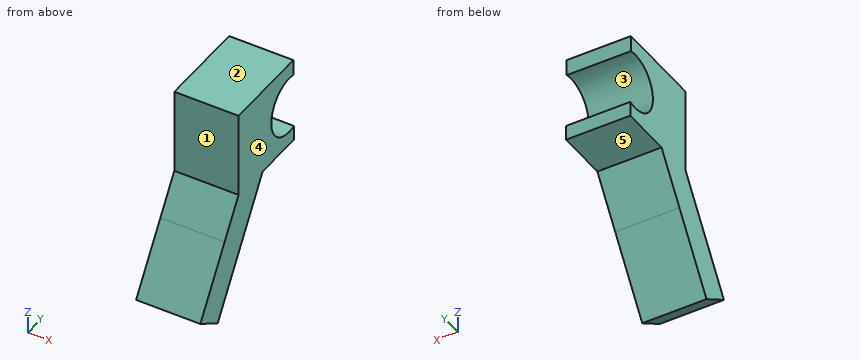
from build123d import *

# Parameters (mm, degrees)
F1_DEPTH = 17.78


with BuildPart() as f1:
    # F0 (on Right) → F1 (new body, symmetric)
    with BuildSketch(Plane.YZ):
        with BuildLine():
            Line((-67.38431, -34.472395), (-51.495798, -44.68644))
            Line((-51.495798, -44.68644), (-26.808784, -6.284426))
            Line((-26.808784, -6.284426), (-10.501343, 19.082699))
            Line((-10.501343, 19.082699), (18.016437, 19.082699))
            Line((18.016437, 19.082699), (18.016437, 27.379308))
            ThreePointArc((18.016437, 27.379308), (-2.608516, 42.469), (17.44899, 58.305159))
            Line((17.44899, 58.305159), (17.44899, 67.38431))
            Line((17.44899, 67.38431), (-32.492471, 67.38431))
            Line((-32.492471, 67.38431), (-32.492471, 19.803789))
            Line((-32.492471, 19.803789), (-45.22348, 0))
            Line((-45.22348, 0), (-67.38431, -34.472395))
        make_face()
    extrude(amount=F1_DEPTH, both=True)


solid = f1.part
Source: CAD feature listing. Evaluate the final solid. Frame: model axes, mm. Face numbers are marked on the shaded views. A direction names the side the tool comes from. Coordinates: 2 decimals unless noted, no trailing zeros. Loops run counter-clockwise (first coordinate to the right, second up) from the corner with the lowest first, then second, coordinate; pieces in that order, holes last. Notation, with made-up numbers: (-12.75, 6.5) - (-6.75, 6.5) arc R27 cw to (-6.75, 41.5) - close; hole circle Ø1 at (59.5, 22). An arc over 180 degrees is marked (long way). Return JSON: item names as keys, results as strings.
Q1. Access query for the marked faces 4 and 5. Directions: +Z, -Z, +X, -X, +Y, -Y. A direction counts if a zero-diameter tool reaches every point of the face in a straight line with its end or side. Return the directions, or none.
Results:
{"face 4": "+Z, -Z, +X, +Y, -Y", "face 5": "-Z, +X, -X, +Y"}
Q2. Material intervals for line 1 along Y through (x, z) = (-0.5, 62); line 2 along Z through (x, y) = (3, 14.5); line 3 along Z through (x, y) = (14, -4.5), sorted ascending.
Results:
{"line 1": "-32.49 to 17.45", "line 2": "19.08 to 26.75, 58.78 to 67.38", "line 3": "19.08 to 67.38"}
Q3. Mould query, pull axis Y, two halves, no side actions, for the marked faces 1, 2 and 3. Classes: released by +Y, released by -Y, zero draft, split by the parting line, or undercut.
Results:
{"face 1": "released by -Y", "face 2": "zero draft", "face 3": "undercut"}
Q4. Section B-B, the plane x = 9.5. Return loops of the section in (y, z), plus the area to 3 significant figures.
Results:
{"outline": "(-67.38, -34.47) - (-51.5, -44.69) - (-10.5, 19.08) - (18.02, 19.08) - (18.02, 27.38) arc R16.05 cw (long way) to (17.45, 58.31) - (17.45, 67.38) - (-32.49, 67.38) - (-32.49, 19.8) - close", "area": "3,200 mm2"}
Q5. Section C-C, the plane z = 60.5. Return loops of the section in (x, y).
Results:
{"outline": "(-17.78, -32.49) - (17.78, -32.49) - (17.78, 17.45) - (-17.78, 17.45) - close"}
Q6. Contact query for flat-ended pins moving along their axis: P1, Ø1, axis at x = -9, y = -30.5, coming from the -Z side; P2, Ø5, axis at x = -9, z = 35.5, coming from the -Y side; P3, Ø8, axis at x = 4.5, z = 16.5, coming from the -Y side; P4, Ø19.5, axis at y = 13.44, z = 42.76, coming from the -X side. Output: stop coordinate, or through.
Results:
{"P1": "z = -12.8", "P2": "y = -32.49", "P3": "y = -37.19", "P4": "through"}
Q7. Section A-A, the plane y = 0. Return loops of the section in (x, z).
Results:
{"outline": "(-17.78, 19.08) - (17.78, 19.08) - (17.78, 33.99) - (-17.78, 33.99) - close; (-17.78, 51.54) - (17.78, 51.54) - (17.78, 67.38) - (-17.78, 67.38) - close"}
Q8. Section D-D, the plane y = 11.5. Return loops of the section in (x, z), plus the area to 3 significant figures.
Results:
{"outline": "(-17.78, 19.08) - (17.78, 19.08) - (17.78, 26.83) - (-17.78, 26.83) - close; (-17.78, 58.7) - (17.78, 58.7) - (17.78, 67.38) - (-17.78, 67.38) - close", "area": "584 mm2"}
